from build123d import *

# Parameters (mm, degrees)
DODANIE_WYCI_GNI_CIE1_DEPTH      = 1.5
DODANIE_WYCI_GNI_CIE1_DEPTH_BACK = 0.5
SZKIC2_R                         = 2
WYTNIJ_WYCI_GNI_CIE1_DEPTH       = 13.403470929


with BuildPart() as part:
    # Szkic1 → Dodanie-wyciągnięcie1 (new body, two sides)
    with BuildSketch(Plane(origin=(91.00215608, -464.566516042, 0), x_dir=(-0.981349358, -0.192232768, 0), z_dir=(0.192232768, -0.981349358, 0))) as dodanie_wyci_gni_cie1_sk:
        with BuildLine():
            Line((-852.646385939, -589.810571865), (-898.412669563, -587.572467385))
            ThreePointArc((-898.412669563, -587.572467385), (-907.277284225, -577.338883089), (-897.89920424, -567.573676668))
            Line((-897.89920424, -567.573676668), (-852.132920616, -569.811781148))
            add(Edge.make_bspline(
                [(-852.646385939, -589.810571865), (-859.599431487, -584.423041675), (-860.017825744, -575.312195542), (-852.132920616, -569.811781148)],
                knots=[-0.289090194, -0.289090194, -0.289090194, -0.289090194, 0.984325659, 0.984325659, 0.984325659, 0.984325659], degree=3, weights=[1.203316353, 0.837838315, 0.76726036, 0.991582488]))
        make_face()
    extrude(amount=DODANIE_WYCI_GNI_CIE1_DEPTH)
    extrude(dodanie_wyci_gni_cie1_sk.sketch, amount=-DODANIE_WYCI_GNI_CIE1_DEPTH_BACK)

    # Szkic2 → Wytnij-wyciągnięcie1 (cut, through all)
    with BuildSketch(Plane(origin=(91.290505232, -466.038540079, 0), x_dir=(-0.981349358, -0.192232768, 0), z_dir=(0.192232768, -0.981349358, 0))):
        with Locations((-901.117736464, -577.428231407)):
            Circle(SZKIC2_R)
    extrude(amount=-WYTNIJ_WYCI_GNI_CIE1_DEPTH, mode=Mode.SUBTRACT)


solid = part.part
Here's how the part is built. I have some questions about the finished solid (model axes, mm). Give positions to 0.01 mm unless a question says otherwise; leave off trailing zeros. Write each loop counter-clockwise with the first axis right and the second up, starting at its lowest first coordinate (ties: lowest second). Pieces come first, ordered by that corner, then holes. Notation, with made-up numbers: (70.5, 67) -> (110.5, 67) arc R17 ccw to (110.5, 99) -> close; hole circle Ø1 at (-36.5, 20.5). An arc over 180 degrees is marked (long way). Use one line per item in the form item = value. Start each with the question number.
1. Will these pins go through, and if not, where does the flat tip stop? pin 1 Ø4 at (x, z) = (971.5, 572.5) entering from +Y; pin 2 Ø6 at (x, y) = (957.5, -298.5) entering from +Z; pin 3 Ø4 at (x, z) = (960.5, 580) entering from -Y.
2. If I drill on L1, parallel to Z at x = 930, y = -300; L2, parallel to Y at x = 945, z = 573.25; L3, parallel to Z at x = 965, y = -294.75, over which ranges is the centre line in solid material (lowest first)?
3. Thinking about a two-plate mould opening in Z: for faces 1 (the face through (954.211, -297.004, 578.536)), 2 (the face through (981.46, -290.66, 577.55)), 3 (the face through (975.668, -291.797, 575.445)), which applies, +Z half, -Z half, draft (parallel to the pull), parting line (faces both ways), or undercut?
4. Imagine slicing it at B-B on x = 961. List the corners of the cut face in (y, z) for me, plus the area to 3 significant figures.
5. Imagine slicing it at A-A on y = -296.75. List the corners of the cut face in (x, z) for me, plus the area to 3 significant figures.
Entries:
q1.pin_1 = -291.19
q1.pin_2 = 588.47
q1.pin_3 = -296.16
q2.L1 = 569.67 to 572.56, 587.44 to 589.7
q2.L2 = -298.81 to -296.77
q2.L3 = 567.94 to 587.97
q3.face_1 = draft
q3.face_2 = parting line
q3.face_3 = undercut
q4.outline = (-295.67, 568.14) -> (-293.64, 568.12) -> (-293.64, 588.15) -> (-295.67, 588.17) -> close
q4.area = 40.8 mm²
q5.outline = (945.11, 568.92) -> (955.51, 568.42) -> (955.51, 588.44) -> (945.11, 588.94) -> close
q5.area = 208 mm²
